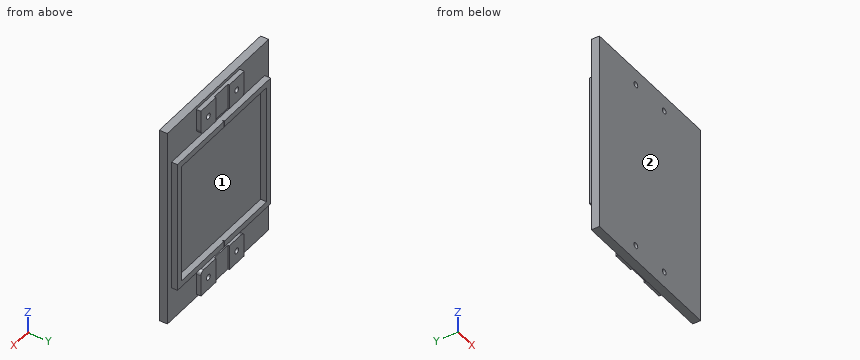
Autodesk Inventor part; units mm, degrees
ref_plane "YZ Plane" through (0, 0, 0) normal (1, 0, 0) x (0, 1, 0)
ref_plane "XZ Plane" through (0, 0, 0) normal (0, 1, 0) x (-1, 0, 0)
ref_plane "XY Plane" through (0, 0, 0) normal (0, 0, 1) x (1, 0, 0)
sketch "Boceto1" plane through (0, 0, 0) normal (0, 1, 0) x (-1, 0, 0)
  line L0 (0, 0) -> (75, 0)
  line L1 (75, 0) -> (75, -100)
  line L2 (75, -100) -> (0, -100)
  line L3 (0, -100) -> (0, 0)
  line L4 (6, -80) -> (69, -80)
  line L5 (69, -80) -> (69, -20)
  line L6 (69, -20) -> (6, -20)
  line L7 (6, -20) -> (6, -80)
  line L8 (6, -80) -> (69, -20) construction
  line L9 (69, -80) -> (6, -20) construction
  line L10 (72, -17) -> (72, -83)
  line L11 (72, -83) -> (3, -83)
  line L12 (3, -83) -> (3, -17)
  line L13 (3, -17) -> (72, -17)
  line L14 (53.5, -1.5) -> (21.5, -1.5)
  line L15 (21.5, -1.5) -> (21.5, -14)
  line L16 (21.5, -14) -> (53.5, -14)
  line L17 (53.5, -14) -> (53.5, -1.5)
  line L18 (69, -50) -> (6, -50) construction
  line L19 (53.5, -7.75) -> (48, -7.75) construction
  line L20 (48, -7.75) -> (27, -7.75) construction
  line L21 (27, -7.75) -> (21.5, -7.75) construction
  circle A0 centre (48, -7.75) radius 1.4
  circle A1 centre (27, -7.75) radius 1.4
  line L22 (53.5, -98.5) -> (21.5, -98.5)
  line L23 (21.5, -98.5) -> (21.5, -86)
  line L24 (21.5, -86) -> (53.5, -86)
  line L25 (53.5, -86) -> (53.5, -98.5)
  circle A2 centre (48, -92.25) radius 1.4
  circle A3 centre (27, -92.25) radius 1.4
  line L26 (58.4347, 0) -> (58.4347, -14) construction
  line L27 (68.2, -14.5) -> (75, -14.5) construction
  line L28 (37.5, -20) -> (37.5, -80) construction
  circle A4 centre (48, -92.25) radius 1.4
  line L29 (48, -7.75) -> (27, -7.75)
  line L30 (37.5, -1.5) -> (37.5, 0)
  line L31 (37.5, -1.5) -> (37.5, -50)
  point P0 (37.5, -14)
  point P1 (37.5, -17)
  point P2 (37.5, -98.5)
  point P3 (37.5, -100)
  dimension "d0" = 100
  dimension "d1" = 75
  dimension "d2" = 60
  dimension "d3" = 63
  dimension "d4" = 3
  dimension "d5" = 12.5
  dimension "d6" = 32
  dimension "d8" = 5.5
  dimension "d9" = 5.5
  dimension "d10" = 2.8
  dimension "d11" = 2.8
  dimension "d14" = 14
  dimension "d32" = 1.5
  dimension "d36" = 1.5
extrude "Extrusión1" add sketch "Boceto1" along normal blind 3 contours L13 L10 L11 L12
extrude "Extrusión2" add sketch "Boceto1" against normal blind 4 contours L14 L17 L16 L31 | L31 L16 L15 L14 | L0 L1 L2 L3 | L22 L23 L24 L25
extrude "Extrusión3" add sketch "Boceto1" along normal blind 2.25 contours L14 L17 L16 L31 | L31 L16 L15 L14 | L22 L23 L24 L25
sketch "Boceto2" plane through (0, 2.25, 0) normal (0, 1, 0) x (1, 0, 0)
  line L0 (-53.5, 1.5) -> (-21.5, 1.5)
  line L1 (-37.5, 1.5) -> (-37.5, 14)
  line L2 (-21.5, 14) -> (-53.5, 14)
  line L3 (-32.5, 1.5) -> (-42.5, 1.5)
  line L4 (-42.5, 1.5) -> (-42.5, 14)
  line L5 (-42.5, 14) -> (-32.5, 14)
  line L6 (-32.5, 14) -> (-32.5, 1.5)
  line L7 (-32.5, 1.5) -> (-42.5, 14) construction
  line L8 (-42.5, 1.5) -> (-32.5, 14) construction
  line L9 (-69, 50) -> (-6, 50) construction
  line L10 (-53.5, 98.5) -> (-21.5, 98.5)
  line L11 (-21.5, 86) -> (-53.5, 86)
  line L12 (-42.5, 98.5) -> (-42.5, 86)
  line L13 (-32.5, 86) -> (-32.5, 98.5)
  point P0 (0, 0)
  point P1 (-37.5, 7.75)
  point P2 (-42.5, 98.5)
  point P3 (-42.5, 1.5)
  point P4 (-32.5, 1.5)
  point P5 (-32.5, 14)
  dimension "d22" = 10
extrude "Extrusión4" cut sketch "Boceto2" against normal blind 0.75
extrude "Extrusión5" add sketch "Boceto1" against normal blind 4 contours L6 L5 L4 L7 | L13 L10 L11 L12
sketch "Boceto3" plane through (0, 3, 0) normal (0, 1, 0) x (1, 0, 0)
  line L0 (-37.5, 20) -> (-37.5, 80) construction
  line L1 (-72, 17) -> (-3, 17)
  line L2 (-37.5, 17) -> (-37.5, 83)
  line L3 (-3, 83) -> (-72, 83)
  line L4 (-37.25, 17) -> (-37.75, 17)
  line L5 (-37.75, 17) -> (-37.75, 83)
  line L6 (-37.75, 83) -> (-37.25, 83)
  line L7 (-37.25, 83) -> (-37.25, 17)
  line L8 (-37.25, 17) -> (-37.75, 83) construction
  line L9 (-37.75, 17) -> (-37.25, 83) construction
  point P0 (0, 0)
  point P1 (-37.5, 50)
  point P2 (-37.25, 83)
  point P3 (-37.75, 17)
  dimension "d27" = 0.5
extrude "Extrusión6" cut sketch "Boceto3" against normal blind 0.75
sketch "Boceto4" plane through (-53.5, 0, -1.5) normal (0, 0, 1) x (1, 0, 0)
  line L0 (16.25, 2.25) -> (15.75, 2.25)
  line L1 (21, 1.5) -> (11, 1.5)
  line L2 (-21.5, 0) -> (53.5, 0)
  line L3 (15.75, 2.25) -> (15.75, 3)
fillet "Empalme1" radius 2 4 edges at (-53.5, 1.125, -86) (-21.5, 1.125, -86) (-21.5, 1.125, -14) (-53.5, 1.125, -14)
equation "\"d9\" = d8"
properties part number "Molde 663FBR 0.75mm"
Check sheet for the modelled part. Datum: model origin and axes. Units: mm. Face numbers are marked on the shaded views. Give positions to 0.01 mm unless a question says otherwise; leave off trailing zeros. Order: outer loops, then holes, each group sorted by start corner. A loop starts at its lowest first (then second) coordinate and runs counter-clockwise, first axis right, second up. Notation, with made-up numbers: (86, 74) -> (142, 74) arc R33 cw to (142, 111) -> close; hole circle Ø6 at (26.25, 12). An arc over 180 degrees is marked (long way). Use CSV: the item, a comma, the result in double quotes. Start each with the question number.
1) Go/stop test with flat-tipped pins: P1, Ø2.5, axis at x = -27, z = -92.25, coming from the -Y side; P2, Ø2, axis at x = -65.5, z = -77.5, coming from the +Y side; P3, Ø0.8, axis at y = 3, z = -18, coming from the -X side; P4, Ø12, axis at x = -24.5, z = -91.5, coming from the +Y side. Record where each tip stops, or that it passes through.
2) Sectioned sample at C-C, the plane z = -29. Record the boundary of the cut face in (x, y), plus the area to 3 significant figures.
3) Sectioned sample at B-B, the plane z = -92.25. Record the boundary of the cut face in (x, y), plus the area to 4 significant figures.
4) Mould release check, pull along Z, two halves, no side actions. Record for the marked faces 1 and 2: released by +Z, released by -Z, zero draft, split by the parting line, or undercut.
5) Sectioned sample at A-A, the plane x = -27. Record the boundary of the cut face in (y, z), plus the area to 3 significant figures.
6) Sectioned sample at D-D, the plane x = -41. Record the boundary of the cut face in (y, z), plus the area to 4 significant figures.
7) Material ranges on line 1 (Z direction, x = -48, y = 0.5); line 2 (Z direction, x = -51.5, y = 1.5); line 3 (Z direction, x = -27, y = -0.5), recorded low to high. Write a range as from..to.
Recorded:
1,P1,"through"
1,P2,"y = 0"
1,P3,"x = -72"
1,P4,"y = 2.25"
2,outline,"(-75, -4) -> (0, -4) -> (0, 0) -> (-3, 0) -> (-3, 3) -> (-6, 3) -> (-6, 0) -> (-69, 0) -> (-69, 3) -> (-72, 3) -> (-72, 0) -> (-75, 0) -> close"
2,area,"318 mm2"
3,outline,"(-75, -4) -> (-49.4, -4) -> (-49.4, 2.25) -> (-53.5, 2.25) -> (-53.5, 0) -> (-75, 0) -> close; (-46.6, -4) -> (-28.4, -4) -> (-28.4, 2.25) -> (-32.5, 2.25) -> (-32.5, 1.5) -> (-42.5, 1.5) -> (-42.5, 2.25) -> (-46.6, 2.25) -> close; (-25.6, -4) -> (0, -4) -> (0, 0) -> (-21.5, 0) -> (-21.5, 2.25) -> (-25.6, 2.25) -> close"
3,area,"329.5 mm2"
4,face 1,"undercut"
4,face 2,"zero draft"
5,outline,"(-4, -100) -> (0, -100) -> (0, -98.5) -> (2.25, -98.5) -> (2.25, -93.65) -> (-4, -93.65) -> close; (-4, -90.85) -> (2.25, -90.85) -> (2.25, -86) -> (0, -86) -> (0, -83) -> (3, -83) -> (3, -80) -> (0, -80) -> (0, -20) -> (3, -20) -> (3, -17) -> (0, -17) -> (0, -14) -> (2.25, -14) -> (2.25, -9.15) -> (-4, -9.15) -> close; (-4, -6.35) -> (2.25, -6.35) -> (2.25, -1.5) -> (0, -1.5) -> (0, 0) -> (-4, 0) -> close"
5,area,"439 mm2"
6,outline,"(-4, -100) -> (0, -100) -> (0, -98.5) -> (1.5, -98.5) -> (1.5, -86) -> (0, -86) -> (0, -83) -> (3, -83) -> (3, -80) -> (0, -80) -> (0, -20) -> (3, -20) -> (3, -17) -> (0, -17) -> (0, -14) -> (1.5, -14) -> (1.5, -1.5) -> (0, -1.5) -> (0, 0) -> (-4, 0) -> close"
6,area,"455.5 mm2"
7,line 1,"-98.5..-93.65, -90.85..-86, -83..-80, -20..-17, -14..-9.15, -6.35..-1.5"
7,line 2,"-98.5..-86, -83..-80, -20..-17, -14..-1.5"
7,line 3,"-100..-93.65, -90.85..-9.15, -6.35..0"
